from build123d import *

# Parameters (mm, degrees)
SKETCH1_R           = 1.5
BOSS_EXTRUDE1_DEPTH = 3


with BuildPart() as part:
    # Sketch1 → Boss-Extrude1 (new body)
    with BuildSketch(Plane(origin=(0, 0, 0), x_dir=(1, 0, 0), z_dir=(0, 1, 0))):
        with BuildLine():
            Line((-9.012614242, -8.062715867), (-27.10951678, -15.558698335))
            ThreePointArc((-27.10951678, -15.558698335), (-32.335768639, -13.393913934), (-30.170984238, -8.167662075))
            Line((-30.170984238, -8.167662075), (-14.527279952, -1.687827594))
            ThreePointArc((-14.527279952, -1.687827594), (-14.532365143, -1.643468323), (-14.537314884, -1.599093734))
            ThreePointArc((-14.537314884, -1.599093734), (-13.375367561, -0.916420891), (-12.08056518, -0.542722374))
            ThreePointArc((-12.08056518, -0.542722374), (-12.092750003, -1.6e-08), (-12.080565181, 0.542722343))
            ThreePointArc((-12.080565181, 0.542722343), (-13.375367564, 0.91642086), (-14.537314887, 1.599093703))
            ThreePointArc((-14.537314887, 1.599093703), (-14.499881093, 1.908945545), (-14.455843804, 2.217928021))
            ThreePointArc((-14.455843804, 2.217928021), (-13.156800144, 2.576605254), (-11.80939679, 2.602450787))
            ThreePointArc((-11.80939679, 2.602450787), (-11.680699543, 3.129833994), (-11.528463026, 3.650909874))
            ThreePointArc((-11.528463026, 3.650909874), (-12.682425794, 4.346994439), (-13.628091988, 5.307139865))
            ThreePointArc((-13.628091988, 5.307139865), (-13.511738162, 5.596745183), (-13.389230858, 5.883801647))
            ThreePointArc((-13.389230858, 5.883801647), (-12.041618538, 5.89404001), (-10.733437524, 5.570271228))
            ThreePointArc((-10.733437524, 5.570271228), (-10.472628711, 6.046374991), (-10.190715165, 6.51029393))
            ThreePointArc((-10.190715165, 6.51029393), (-11.125197663, 7.48132753), (-11.790137141, 8.653513216))
            ThreePointArc((-11.790137141, 8.653513216), (-11.602792603, 8.903135886), (-11.410163954, 9.148703915))
            ThreePointArc((-11.410163954, 9.148703915), (-10.105820527, 8.80980568), (-8.926012227, 8.158486891))
            ThreePointArc((-8.926012227, 8.158486891), (-8.550865537, 8.550865523), (-8.158486906, 8.926012214))
            ThreePointArc((-8.158486906, 8.926012214), (-8.809805695, 10.105820514), (-9.148703931, 11.410163942))
            ThreePointArc((-9.148703931, 11.410163942), (-8.903135901, 11.602792591), (-8.653513232, 11.79013713))
            ThreePointArc((-8.653513232, 11.79013713), (-7.481327547, 11.125197652), (-6.510293947, 10.190715155))
            ThreePointArc((-6.510293947, 10.190715155), (-6.046375007, 10.472628701), (-5.570271245, 10.733437515))
            ThreePointArc((-5.570271245, 10.733437515), (-5.894040027, 12.04161853), (-5.883801664, 13.38923085))
            ThreePointArc((-5.883801664, 13.38923085), (-5.5967452, 13.511738155), (-5.307139882, 13.628091982))
            ThreePointArc((-5.307139882, 13.628091982), (-4.346994456, 12.682425788), (-3.650909891, 11.52846302))
            ThreePointArc((-3.650909891, 11.52846302), (-3.129834011, 11.680699538), (-2.602450802, 11.809396786))
            ThreePointArc((-2.602450802, 11.809396786), (-2.57660527, 13.156800141), (-2.217928037, 14.455843802))
            ThreePointArc((-2.217928037, 14.455843802), (-1.908945561, 14.499881091), (-1.599093718, 14.537314885))
            ThreePointArc((-1.599093718, 14.537314885), (-0.916420875, 13.375367563), (-0.542722359, 12.08056518))
            ThreePointArc((-0.542722359, 12.08056518), (2e-09, 12.092750003), (0.542722362, 12.08056518))
            ThreePointArc((0.542722362, 12.08056518), (0.916420879, 13.375367562), (1.599093721, 14.537314885))
            ThreePointArc((1.599093721, 14.537314885), (1.908945564, 14.49988109), (2.21792804, 14.455843801))
            ThreePointArc((2.21792804, 14.455843801), (2.576605273, 13.15680014), (2.602450806, 11.809396786))
            ThreePointArc((2.602450806, 11.809396786), (3.129834014, 11.680699537), (3.650909894, 11.528463019))
            ThreePointArc((3.650909894, 11.528463019), (4.346994459, 12.682425786), (5.307139885, 13.628091981))
            ThreePointArc((5.307139885, 13.628091981), (5.596745203, 13.511738153), (5.883801667, 13.389230849))
            ThreePointArc((5.883801667, 13.389230849), (5.89404003, 12.041618528), (5.570271248, 10.733437514))
            ThreePointArc((5.570271248, 10.733437514), (6.04637501, 10.4726287), (6.510293949, 10.190715153))
            ThreePointArc((6.510293949, 10.190715153), (7.481327549, 11.12519765), (8.653513234, 11.790137128))
            ThreePointArc((8.653513234, 11.790137128), (8.903135904, 11.602792589), (9.148703933, 11.41016394))
            ThreePointArc((9.148703933, 11.41016394), (8.809805697, 10.105820513), (8.158486908, 8.926012212))
            ThreePointArc((8.158486908, 8.926012212), (8.550865539, 8.550865522), (8.926012229, 8.15848689))
            ThreePointArc((8.926012229, 8.15848689), (10.105820529, 8.809805679), (11.410163956, 9.148703914))
            ThreePointArc((11.410163956, 9.148703914), (11.602792604, 8.903135884), (11.790137143, 8.653513214))
            ThreePointArc((11.790137143, 8.653513214), (11.125197664, 7.481327529), (10.190715166, 6.510293928))
            ThreePointArc((10.190715166, 6.510293928), (10.472628712, 6.046374989), (10.733437525, 5.570271227))
            ThreePointArc((10.733437525, 5.570271227), (12.041618538, 5.894040009), (13.389230858, 5.883801646))
            ThreePointArc((13.389230858, 5.883801646), (13.511738162, 5.596745182), (13.628091989, 5.307139864))
            ThreePointArc((13.628091989, 5.307139864), (12.967370885, 4.588201714), (12.187984486, 3.999999979))
            Line((12.187984486, 3.999999979), (11.544422781, 3.600125731))
            ThreePointArc((11.544422781, 3.600125731), (5.967242425, -10.517919019), (-9.012614242, -8.062715867))
        make_face()
        Circle(SKETCH1_R, mode=Mode.SUBTRACT)
        with Locations((-28.640250509, -11.863180205)):
            Circle(SKETCH1_R, mode=Mode.SUBTRACT)
        with Locations((-6.929096489, -2.870125744)):
            Circle(SKETCH1_R, mode=Mode.SUBTRACT)
        with Locations((6.929111486, 2.870131956)):
            Circle(SKETCH1_R, mode=Mode.SUBTRACT)
    extrude(amount=BOSS_EXTRUDE1_DEPTH)


solid = part.part
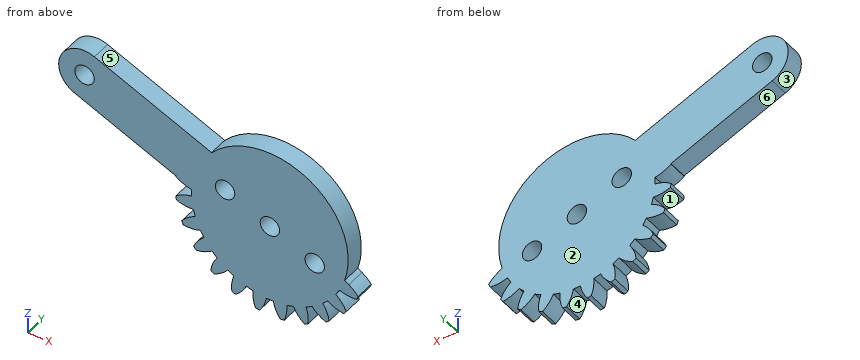
Can you work these out from the model? Positions are in its coordinate system, mm. Face numbers are marked on the shaded views. A direction names the side the tool comes from. Give positions to 0.01 mm unless a question says otherwise; leave off trailing zeros. Write each loop counter-clockwise with the first axis right and the second up, starting at its lowest first coordinate (ties: lowest second). Pieces come first, ordered by that corner, then holes. Notation, with made-up numbers: M -14.5,31.25 L 41.5,31.25 A28 ccw 41.5,63.25 Z; hole C -2,-12 d8. An arc over 180 degrees is marked long. Answer in a Markdown table with one row per item. Add a question column.
Item 1: Imagine slicing it at A-A, the plane z = 0. Write out the boundary of the cut face in (x, y).
Item 2: Imagine slicing it at B-B, the plane x = 0. Write out the boundary of the cut face in (y, z), plus the area to 3 significant figures.
Item 3: We'd pull the mould along Z, two halves only. Please class the marked faces 1, 2 and 3: released by +Z, released by -Z, zero draft, split by the parting line, or undercut.
Item 4: On a 3-axis mill with a long thin cutter (end or side, diameter ignored), from which of +Z, -Z, +X, -X, +Y, -Y can I reach the whole of each face in a straight line? I mean the marked faces 4, 5 and 6. Say none if no direction works.
Item 5: Imagine slicing it at C-C, the plane x = -16. Write out the boundary of the cut face in (y, z), plus the area to 3 significant figures.
Item 6: Imagine slicing it at D-D, the plane y = 2.2. State how many separate pieces and enclosed holes the cut face has, plus the area to 3 significant figures.
Item 7: For pin 1 Ø4 at (x, z) = (-23.5, 5) entering from -Y, with a flat end and sliding along its axis, tell me the tip position at first contact or that it passes through.
Item 8: Please list where these lines run through material, in increasing order: L1, parallel to X at y = 0.1, z = -13; L2, parallel to X at y = 2.7, z = -12.5; L3, parallel to X at y = 0.8, z = -11.
Evaluation:
| question | item | result |
|---|---|---|
| 1 | outline | M -12.09,0 L -1.5,0 L -1.5,3 L -12.09,3 Z; M 1.5,0 L 12.09,0 L 12.09,3 L 1.5,3 Z |
| 2 | outline | M 0,-12.09 L 3,-12.09 L 3,-1.5 L 0,-1.5 Z; M 0,1.5 L 3,1.5 L 3,12.09 L 0,12.09 Z |
| 2 | area | 63.6 mm² |
| 3 | face 1 | undercut |
| 3 | face 2 | zero draft |
| 3 | face 3 | split by the parting line |
| 4 | face 4 | -Z, +Y, -Y |
| 4 | face 5 | +Z, +Y, -Y |
| 4 | face 6 | -Z, -X, +Y, -Y |
| 5 | outline | M 0,2.3 L 3,2.3 L 3,10.96 L 0,10.96 Z |
| 5 | area | 26.0 mm² |
| 6 | separate pieces | 1 |
| 6 | enclosed holes | 4 |
| 6 | area | 654 mm² |
| 7 | pin 1 | stops at y = 0 |
| 8 | L1 | x = -5.92 to -4.62, -2.6 to -0.77, 0.77 to 2.6, 4.62 to 5.92 |
| 8 | L2 | x = -5.93 to -4.21, -2.63 to -0.63, 0.63 to 2.63, 4.21 to 5.93 |
| 8 | L3 | x = -9.08 to -7.32, -5.67 to 5.67, 7.32 to 9.08 |
